Geometry: see drawing. Coordinates: mm, zero at the bounding-box minimum. A direction names the side the tool comes from. Give positions to 0.01 mm unless a question says otherwise; leave off trailing zeros. Write each loop counter-clockwise with the first axis right and the second up, starting at its lowest first coordinate (ties: lowest second). Pieces come first, ordered by that corner, then holes. Notation, with made-up numbers: M -39,21.5 L 13,21.5 A25 ccw 13,33.5 Z; hole C -14,-15.5 d8. An arc over 180 degrees is marked long. Use a Markdown table: item, result. Add a question column.
1) Pin query (flat end, axial travel): pin 1 (3 mm diameter, centred on y = 3.5, z = 7, fed in from +X); pin 2 (1.9 mm diameter, centred on x = 80.5, y = 2.5, fed in from -Z); pin 3 (1.9 mm diameter, centred on y = 3, z = 5.5, fed in from -X). Return the tip coordinate at first contact, or that it passes through.
2) Set-up query: the marked faces 1, 2 and 3. Return all of +Z, -Z, +X, -X, +Y, -Y with unobstructed straight access to the full face (end or side cutting, diameter ignored); none if empty.
3) Section B-B on z = 5.5. Return the cut outline in (x, y).
4) Section A-A on y = 2.5. Return the cut outline in (x, z).
5) Line query: line 1 (Z direction, x = 4, y = 6.25); line 2 (X direction, y = 2, z = 45). Output: solid intervals per line, ascending.
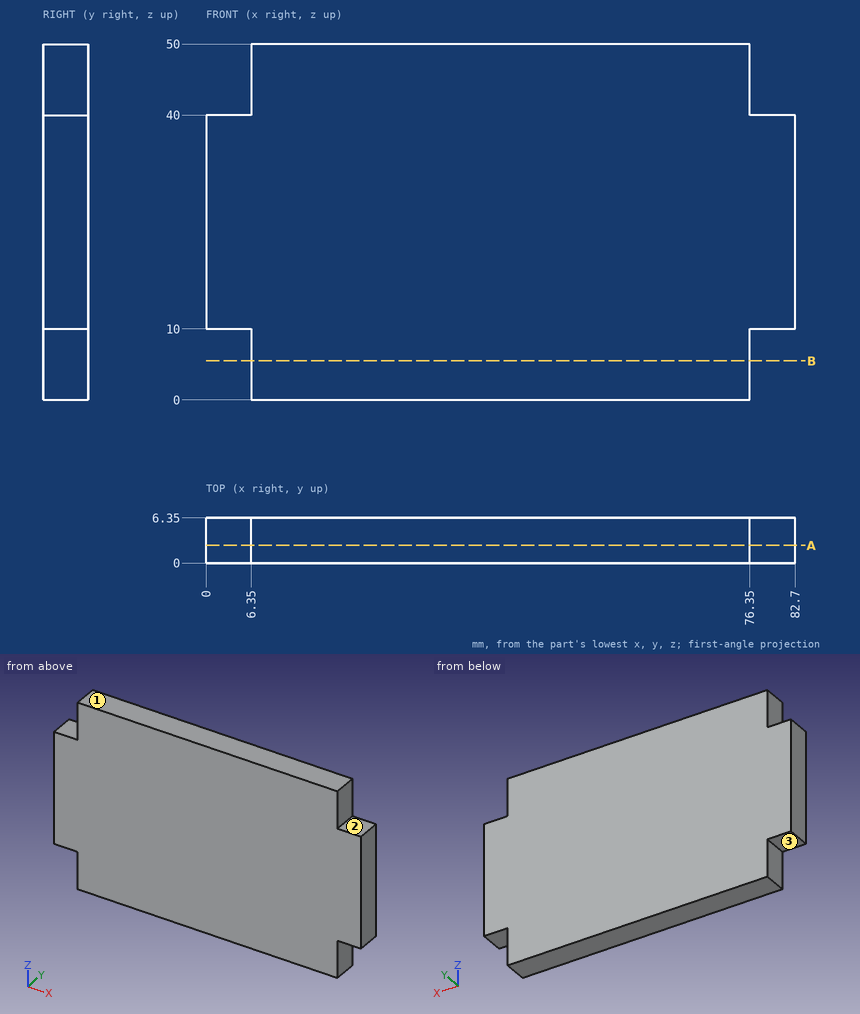
Found:
| question | item | result |
|---|---|---|
| 1 | pin 1 | x = 76.35 |
| 1 | pin 2 | z = 10 |
| 1 | pin 3 | x = 6.35 |
| 2 | face 1 | +Z, +X, -X, +Y, -Y |
| 2 | face 2 | +Z, +X, +Y, -Y |
| 2 | face 3 | -Z, -X, +Y, -Y |
| 3 | outline | M 6.35,0 L 76.35,0 L 76.35,6.35 L 6.35,6.35 Z |
| 4 | outline | M 0,10 L 6.35,10 L 6.35,0 L 76.35,0 L 76.35,10 L 82.7,10 L 82.7,40 L 76.35,40 L 76.35,50 L 6.35,50 L 6.35,40 L 0,40 Z |
| 5 | line 1 | 10 to 40 |
| 5 | line 2 | 6.35 to 76.35 |
